from build123d import *

# Parameters (mm, degrees)
F0_R     = 14.2875
F1_DEPTH = 2.286


with BuildPart() as f1:
    # F0 (on Top) → F1 (new body)
    with BuildSketch(Plane.XY):
        with BuildLine():
            ThreePointArc((-8.360123, -122.495806), (6.386198, -113.716984), (12.183869, -97.564316))
            ThreePointArc((12.183869, -97.564316), (0.052198, -75.905335), (-24.754041, -74.936089))
            ThreePointArc((-24.754041, -74.936089), (-34.875112, -84.295987), (-38.616131, -97.564316))
            Line((-38.616131, -97.564316), (-38.594074, -96.545842))
            ThreePointArc((-38.594074, -96.545842), (-31.353941, -114.860812), (-13.200028, -122.495806))
            Line((-13.200028, -122.495806), (-13.176682, -122.495806))
            Line((-13.176682, -122.495806), (-8.360123, -122.495806))
        make_face()
        with Locations((-13.216131, -97.564316)):
            Circle(F0_R, mode=Mode.SUBTRACT)
        with BuildLine():
            ThreePointArc((-24.754041, -74.936089), (0.052198, -75.905335), (12.183869, -97.564316))
            ThreePointArc((12.183869, -97.564316), (6.386198, -113.716984), (-8.360123, -122.495806))
            Line((-8.360123, -122.495806), (148.645369, -122.495806))
            Line((148.645369, -122.495806), (148.645369, -97.564316))
            ThreePointArc((148.645369, -97.564316), (140.703649, -47.485912), (117.657808, -2.321693))
            Line((117.657808, -2.321693), (-24.754041, -74.936089))
        make_face()
        with BuildLine():
            ThreePointArc((-8.866676, -122.589148), (-8.613163, -122.543761), (-8.360123, -122.495806))
            Line((-8.360123, -122.495806), (-13.176682, -122.495806))
            Line((-13.176682, -122.495806), (-8.866676, -122.589148))
        make_face()
        with BuildLine():
            Line((-38.594074, -96.545842), (-38.616131, -97.564316))
            ThreePointArc((-38.616131, -97.564316), (-29.566725, -117.001859), (-8.866676, -122.589148))
            Line((-8.866676, -122.589148), (-13.176682, -122.495806))
            Line((-13.176682, -122.495806), (-13.200028, -122.495806))
            ThreePointArc((-13.200028, -122.495806), (-31.353941, -114.860812), (-38.594074, -96.545842))
        make_face()
        with BuildLine():
            Line((118.499122, -1.892715), (117.657808, -2.321693))
            ThreePointArc((117.657808, -2.321693), (140.703649, -47.485912), (148.645369, -97.564316))
            Line((148.645369, -97.564316), (148.645369, -122.495806))
            Line((148.645369, -122.495806), (148.708869, -122.495806))
            ThreePointArc((148.708869, -122.495806), (153.198997, -120.635934), (155.058869, -116.145806))
            Line((155.058869, -116.145806), (155.058869, -97.564316))
            ThreePointArc((155.058869, -97.564316), (147.803234, -48.684465), (126.662021, -4.01979))
            ThreePointArc((126.662021, -4.01979), (122.984803, -1.404965), (118.499122, -1.892715))
        make_face()
    extrude(amount=F1_DEPTH)


solid = f1.part
Geometry check sheet. Reference: the model listing, model coordinates, mm. Round coordinates to 2 decimals unless told otherwise and drop trailing zeros. Loops run counter-clockwise (first coordinate to the right, second up) from the corner with the lowest first, then second, coordinate; pieces in that order, holes last. Notation, with made-up numbers: (-25, 58.25) -> (19, 58.25) arc R9 ccw to (19, 75.25) -> close; hole circle Ø6 at (32, 28.25). An arc over 180 degrees is marked (long way). Answer as a JSON object with one key per item and string values. Group by question number.
Item 1: Cross-section at B-B, the plane y = -88. Record the cut outline in (x, z).
Item 2: Thickness scan on line 1 along X through (y, z) = (-98.5, 0.7); line 2 along X through (y, z) = (-107, 0.4); line 3 along X through (y, z) = (-44, 1.75). Record the ranges inside material, lowest first.
Item 3: Depth check by flat-ended pin: pin 1 Ø1 at (y, z) = (-63.5, 0.5) entering from -X. Enter the tip coordinate at first touch or a pass-through.
Item 4: Cross-section at D-D, the plane y = -25.5. Record the cut outline in (x, z), plus the area to 3 significant figures.
Item 5: Release check for a two-part mould opening along X. For faces 1 (the face through (153.149, -120.685, 1.127)), 2 (the face through (78, -75, 2.286)), 3 (the face through (-16.313, -111.512, 1.127)) record: pulls with the +X half, pulls with the -X half, needs draft (parallel to the pull), parting line crosses it, or undercut.
Item 6: Cross-section at C-C, the plane x = -22.5. Record the cut outline in (y, z).
Determined:
{
 "1": {"outline": "(-36.75, 0) -> (-23.83, 0) -> (-23.83, 2.29) -> (-36.75, 2.29) -> close; (-2.6, 0) -> (154.79, 0) -> (154.79, 2.29) -> (-2.6, 2.29) -> close"},
 "2": {"line 1": "x = -38.6 to -27.47, 1.04 to 155.06", "line 2": "x = -36.8 to -23.94, -2.49 to 155.06", "line 3": "x = 35.92 to 146.31"},
 "3": {"pin 1": "stops at x = -3.31"},
 "4": {"outline": "(72.2, 0) -> (138.85, 0) -> (138.85, 2.29) -> (72.2, 2.29) -> close", "area": "152 mm²"},
 "5": {"face 1": "pulls with the +X half", "face 2": "needs draft", "face 3": "undercut"},
 "6": {"outline": "(-121.21, 0) -> (-108.42, 0) -> (-108.42, 2.29) -> (-121.21, 2.29) -> close; (-86.7, 0) -> (-73.79, 0) -> (-73.79, 2.29) -> (-86.7, 2.29) -> close"}
}
